Job drawing, mm, ordinate dimensions from the low corner. One solid piece. A direction names the side the tool comes from. Round coordinates to 2 decimals unless told otherwise and drop trailing zeros. Order: outer loops, then holes, each group sorted by start corner. A loop starts at its lowest first (then second) coordinate and runs counter-clockwise, first axis right, second up. Notation, with made-up numbers: M 83,69.5 L 111,69.5 A19 cw 111,83.5 Z; hole C 54.25,52 d8. An arc over 180 degrees is marked long. Answer as a JSON object with one key per item and string values. Group by question number.
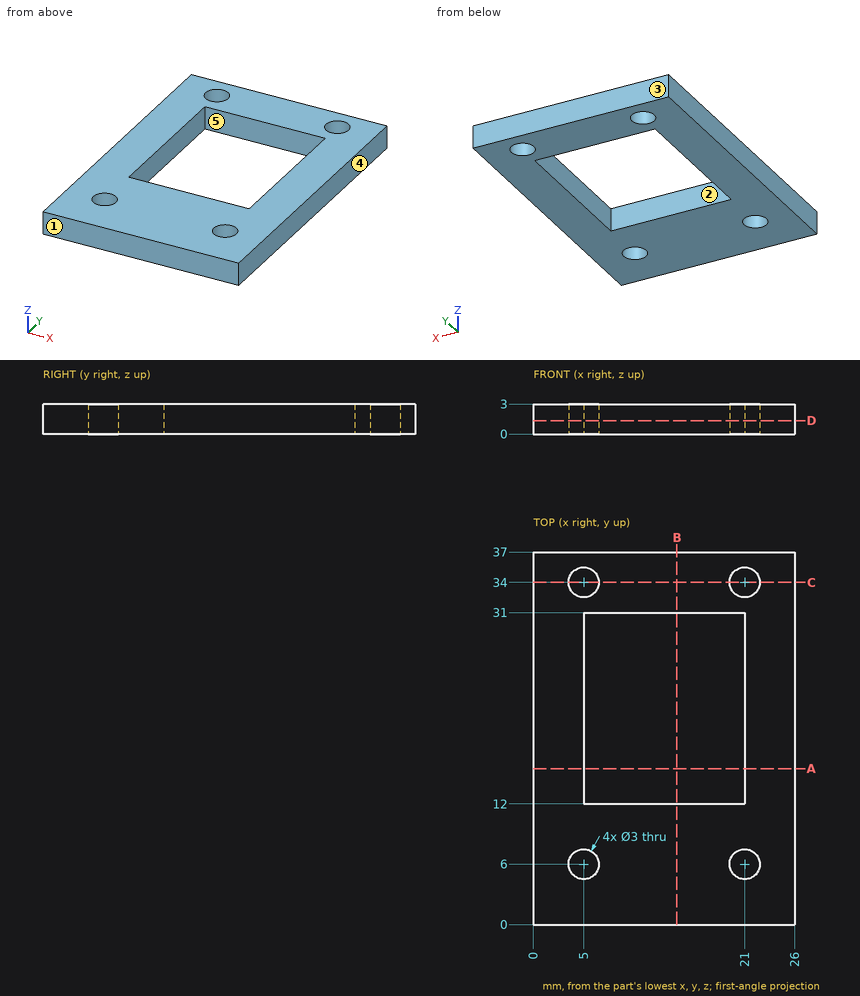
Item 1: Cut at C-C, the plane y = 34. Give the cut face in (x, z).
Item 2: Cut at D-D, the plane z = 1.35. Give the cut face in (x, y).
Item 3: 3-axis set-ups, long thin cutter, end or side, ignore diameter. For the marked faces 1 and 2: which of +Z, -Z, +X, -X, +Y, -Y reach the whole face in a straight line?
Item 4: Two-plate mould, pull along Y, no slides. Class the marked faces 3, 4 and 5: +Y half, -Y half, draft (parallel to the pull), parting line (faces both ways), or undercut.
Item 5: Cut at B-B, the plane x = 14.25. Give the cut face in (y, z).
Item 6: Cut at A-A, the plane y = 15.5. Give the cut face in (x, z), and give its area (3 significant figures).
Item 7: Drill centre lines: line 1 (X direction, y = 34, z = 0.6); line 2 (Y direction, x = 17, z = 1.9); line 3 (X direction, y = 22.5, z = 2.45). Where is each one in solid material? Low to high. Write a range as [from, to].
Response values:
{
 "1": {"outline": "M 0,0 L 3.5,0 L 3.5,3 L 0,3 Z; M 6.5,0 L 19.5,0 L 19.5,3 L 6.5,3 Z; M 22.5,0 L 26,0 L 26,3 L 22.5,3 Z"},
 "2": {"outline": "M 0,0 L 26,0 L 26,37 L 0,37 Z; hole C 5,6 d3; hole C 5,34 d3; hole M 5,12 L 21,12 L 21,31 L 5,31 Z; hole C 21,6 d3; hole C 21,34 d3"},
 "3": {"face 1": "+Z, -Z, +X, -X, -Y", "face 2": "+Z, -Z"},
 "4": {"face 3": "+Y half", "face 4": "draft", "face 5": "undercut"},
 "5": {"outline": "M 0,0 L 12,0 L 12,3 L 0,3 Z; M 31,0 L 37,0 L 37,3 L 31,3 Z"},
 "6": {"outline": "M 0,0 L 5,0 L 5,3 L 0,3 Z; M 21,0 L 26,0 L 26,3 L 21,3 Z", "area": "30.0 mm^2"},
 "7": {"line 1": "[0, 3.5], [6.5, 19.5], [22.5, 26]", "line 2": "[0, 12], [31, 37]", "line 3": "[0, 5], [21, 26]"}
}
